Work out the finished part from the listing and answer in its coordinate system (mm). Face numbers are marked on the shaded views. A direction names the side the tool comes from. Coordinates: 2 decimals unless noted, no trailing zeros. Write each loop counter-clockwise with the first axis right and the second up, starting at its lowest first coordinate (ties: lowest second). Pieces come first, ordered by that corner, then holes. Notation, with made-up numbers: (39.5, 39.25) - (60.5, 39.25) arc R5 ccw to (60.5, 48.25) - close; hole circle Ø4 at (-27, 14.25). An arc over 180 degrees is marked (long way). Use one line per item in the form item = value. Start each with the question number.
Item 1: A cutting plane is placed at D-D (z = 58.5). Write down the section's boundary in (x, y), then the cut area to 3 significant figures.
Item 2: A cutting plane is placed at B-B (z = 45). Write down the section's boundary in (x, y), then the cut area to 3 significant figures.
Item 3: Consider probe 1 along Y at (x, z) = (-40, 53); probe 2 along X at (y, z) = (-19, 45); probe 3 along Z at (x, y) = (-23.5, -18.5). Determine where each line is inside the solid, lowest interval first.
Item 4: Given pin 1 (1.5 mm diameter, centred on x = -74.5, z = 30, fed in from -Y); pin 2 (8 mm diameter, centred on y = -32, z = 50.5, fed in from +X); pin 3 (1 mm diameter, centred on y = -27, z = 59.5, fed in from +X), each flat-ended and moving along its own axis, determine where each tip first touches the part or whether it passes through.
Item 5: For the marked faces 4 and 5, determine the directions among +Z, -Z, +X, -X, +Y, -Y from which every point of the face is accessible in a straight line to the end or side of a thin tool.
Item 6: Determine the mould class of the marked faces 1, 2 and 3 for opening direction Y: released by +Y, released by -Y, zero draft, split by the parting line, or undercut.
Item 7: A cutting plane is placed at C-C (y = -20). Write down the section's boundary in (x, z).
Item 8: A cutting plane is placed at A-A (x = -38). Write down the section's boundary in (y, z), then the cut area to 3 significant figures.
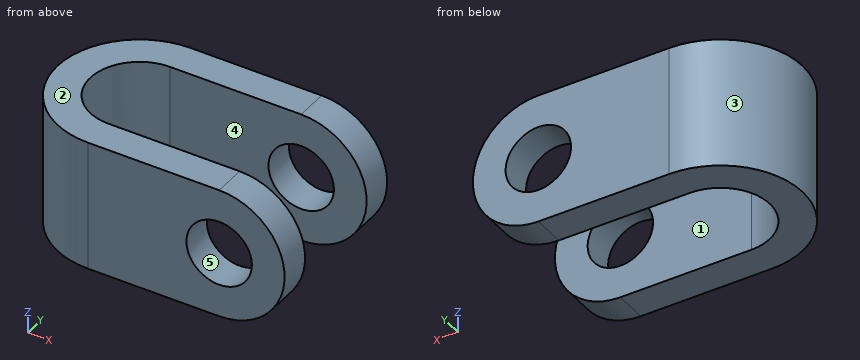
from build123d import *

# Parameters (mm, degrees)
EXTRUDE_THIN1_DEPTH = 90
SKETCH2_R           = 10
BOSS_EXTRUDE1_DEPTH = 90


with BuildPart() as part:
    # Sketch1 → Extrude-Thin1 (new body)
    with BuildSketch(Plane.XY):
        with BuildLine():
            Line((0, -15), (-60, -15))
            ThreePointArc((-60, -15), (-85, -40), (-60, -65))
            Line((-60, -65), (0, -65))
            Line((0, -65), (0, -55))
            Line((0, -55), (-60, -55))
            ThreePointArc((-60, -55), (-75, -40), (-60, -25))
            Line((-60, -25), (0, -25))
            Line((0, -25), (0, -15))
        make_face()
    extrude(amount=EXTRUDE_THIN1_DEPTH)


with BuildPart() as body_2:
    # Sketch2 → Boss-Extrude1 (new body)
    with BuildSketch(Plane(origin=(0, 0, 0), x_dir=(1, 0, 0), z_dir=(0, 1, 0))):
        with BuildLine():
            Line((-85, -25), (-85, -65))
            Line((-85, -65), (-20, -65))
            ThreePointArc((-20, -65), (0, -45), (-20, -25))
            Line((-20, -25), (-85, -25))
        make_face()
        with Locations(Location((-20, -45, 0), (0, 0, 270))):
            Circle(SKETCH2_R, mode=Mode.SUBTRACT)
    extrude(amount=-BOSS_EXTRUDE1_DEPTH)


with BuildPart() as part_1:
    add(part.part)

    # Combine 1: intersect body 2
    add(body_2.part, mode=Mode.INTERSECT)


solid = part_1.part
Answer:
q1.outline = (-60, -65) - (-5.24, -65) - (-5.24, -55) - (-60, -55) arc R15 cw to (-60, -25) - (-5.24, -25) - (-5.24, -15) - (-60, -15) arc R25 ccw to start
q1.area = 1,720 mm²
q2.outline = (-60, -65) - (-30, -65) - (-30, -55) - (-60, -55) arc R15 cw to (-60, -25) - (-30, -25) - (-30, -15) - (-60, -15) arc R25 ccw to start; (-10, -65) - (0, -65) - (0, -55) - (-10, -55) - close; (-10, -25) - (0, -25) - (0, -15) - (-10, -15) - close
q2.area = 1,430 mm²
q3.probe_1 = -65 to -55, -25 to -15
q3.probe_2 = -73.56 to -30, -10 to 0
q3.probe_3 = 25 to 35.63, 54.37 to 65
q4.pin_1 = -60.88
q4.pin_2 = -69
q4.pin_3 = -66.54
q5.face_4 = +Z, -Z, +X
q5.face_5 = +Y, -Y
q6.face_1 = undercut
q6.face_2 = zero draft
q6.face_3 = split by the parting line
q7.outline = (-75, 25) - (-20, 25) arc R20 ccw to (-20, 65) - (-75, 65) - close; hole circle Ø20 at (-20, 45)
q8.outline = (-65, 25) - (-55, 25) - (-55, 65) - (-65, 65) - close; (-25, 25) - (-15, 25) - (-15, 65) - (-25, 65) - close
q8.area = 800 mm²
